The listing builds one solid part. Answer for the finished solid, in the listing's coordinates (mm). Face numbers are marked on the shaded views. A direction names the side the tool comes from. Round coordinates to 2 decimals unless told otherwise and drop trailing zeros. Order: outer loops, then holes, each group sorted by start corner. A loop starts at its lowest first (then second) coordinate and runs counter-clockwise, first axis right, second up. Notation, with made-up numbers: M 78,85 L 122,85 A19 ccw 122,91 Z; hole C 23,32.5 d9. An arc over 180 degrees is marked long. Put each result on its own line as item: value. Start each with the question number.
1. The part is cut by section B-B (y = 6). Give the vertices of the cut face in (x, z).
2. Each of these flat-tipped pins is pushed along its axis until it touches: pin 1 Ø1.4 at (x, z) = (-1, -1.5) entering from -Y; pin 2 Ø1.8 at (x, y) = (0, 4) entering from +Z; pin 3 Ø1 at (x, y) = (-2.5, 13.5) entering from -Z. Where does it stop, or does it pass through?
3. Which of the six approach directions +Z, -Z, +X, -X, +Y, -Y give full straight-line access (tool end or side, diameter ignored) to the marked faces 1, 2 and 3?
4. Consider line 1 (Y direction, x = 0, z = 4.1) (3 decimals); line 2 (X direction, y = 3.25, z = 0); line 3 (X direction, y = 22.35, z = 0). Determine where each line is inside the solid, lowest interval first.
5. The part is cut by section C-C (x = 1.25). Count the separate pieces of the cut face and the enclosed holes in it, then the cut area to 3 significant figures.
6. The mould has two halves that part along X. Classify the marked faces 4, 5 and 6: +X half, -X half, draft (parallel to the pull), parting line (faces both ways), or undercut.
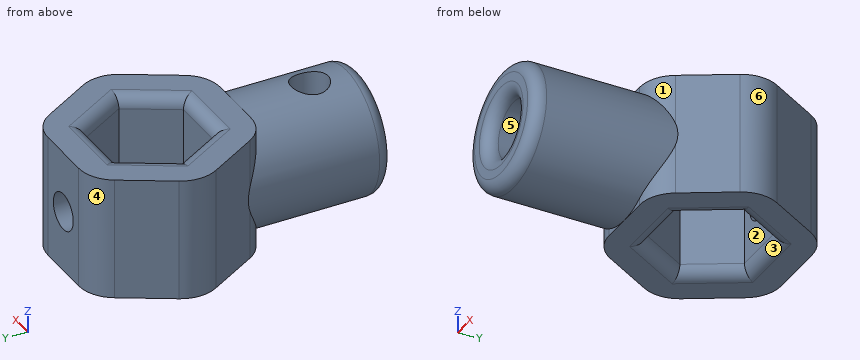
from build123d import *

# Parameters (mm, degrees)
ESBO_O1_R                = 5
ESBO_O1_R_2              = 2.3
RESSALTO_EXTRUS_O1_DEPTH = 12
ESBO_O2_R                = 1.5
CORTE_EXTRUS_O1_DEPTH    = 10
RESSALTO_EXTRUS_O2_DEPTH = 5
ESBO_O4_R                = 1.5
CORTE_EXTRUS_O2_DEPTH    = 5
FILETE1_R                = 1
FILETE2_R                = 3


with BuildPart() as part:
    # Esboço1 → Ressalto-extrusão1 (new body)
    with BuildSketch(Plane(origin=(0, 0, 0), x_dir=(1, 0, 0), z_dir=(0, 1, 0))):
        with Locations(Location((0, 0, 0), (0, 0, 270))):
            Circle(ESBO_O1_R)
        with Locations(Location((0, 0, 0), (0, 0, 270))):
            Circle(ESBO_O1_R_2, mode=Mode.SUBTRACT)
    extrude(amount=RESSALTO_EXTRUS_O1_DEPTH)

    # Esboço2 → Corte-extrusão1 (cut)
    with BuildSketch(Plane.XY):
        with Locations(Location((0, 4, 0), (0, 0, 180))):
            Circle(ESBO_O2_R)
    extrude(amount=CORTE_EXTRUS_O1_DEPTH, mode=Mode.SUBTRACT)

    # Esboço3 → Ressalto-extrusão2 (add, symmetric)
    with BuildSketch(Plane.XY):
        Polygon((4.041451884, 10), (8.082903769, 17), (4.041451884, 24), (-4.041451884, 24), (-8.082903769, 17), (-4.041451884, 10), align=None)
        Polygon((2.309401077, 13), (4.618802154, 17), (2.309401077, 21), (-2.309401077, 21), (-4.618802154, 17), (-2.309401077, 13), align=None, mode=Mode.SUBTRACT)
    extrude(amount=RESSALTO_EXTRUS_O2_DEPTH, both=True)

    # Esboço4 → Corte-extrusão2 (cut)
    with BuildSketch(Plane(origin=(0, 24, 0), x_dir=(1, 0, 0), z_dir=(0, 1, 0))):
        with Locations(Location((0, 0, 0), (0, 0, 270))):
            Circle(ESBO_O4_R)
    extrude(amount=-CORTE_EXTRUS_O2_DEPTH, mode=Mode.SUBTRACT)

    # Filete1
    filete1_edges = [part.edges().sort_by_distance(p)[0] for p in [
        (0, 0, -5),
        (0, 13, -5),
        (3.464101615, 15, -5),
        (3.464101615, 19, -5),
        (0, 21, -5),
        (-3.464101615, 19, -5),
        (-3.464101615, 15, -5),
        (0, 13, 5),
        (3.464101615, 15, 5),
        (3.464101615, 19, 5),
        (0, 21, 5),
        (-3.464101615, 19, 5),
        (-3.464101615, 15, 5),
        (0, 0, -2.3),
    ]]
    fillet(filete1_edges, radius=FILETE1_R - 0.0001)  # a hair under: the kernel refuses the full size

    # Filete2
    filete2_edges = [part.edges().sort_by_distance(p)[0] for p in [
        (-4.041451884, 10, -3.971960144),
        (-4.041451884, 10, 3.971960144),
        (8.082903769, 17, 0),
        (4.041451884, 10, 3.971960144),
        (4.041451884, 10, -3.971960144),
        (4.041451884, 24, 0),
        (-4.041451884, 24, 0),
        (-8.082903769, 17, 0),
    ]]
    fillet(filete2_edges, radius=FILETE2_R)


solid = part.part
Resolved:
1. outline: C 0,0 d10; hole C 0,0 d4.6
2. pin 1: y = 0.4
2. pin 2: z = -2.12
2. pin 3: z = -4.81
3. face 1: +Z, +X, -Y
3. face 2: +Z, -Z
3. face 3: -Z
4. line 1: 0.005 to 2.5, 5.5 to 12.995, 21.005 to 24
4. line 2: -5 to -2.3, 2.3 to 5
4. line 3: -4.99 to -1.5, 1.5 to 4.99
5. separate pieces: 4
5. enclosed holes: 0
5. area: 107 mm2
6. face 4: -X half
6. face 5: undercut
6. face 6: +X half
